Verification items for this drawing (mm, ordinates from the low corner). Round coordinates to 2 decimals unless told otherwise and drop trailing zeros. Order: outer loops, then holes, each group sorted by start corner. A loop starts at its lowest first (then second) coordinate and runs counter-clockwise, first axis right, second up. Notation, with made-up numbers: (25, -6.5) -> (49, -6.5) arc R16 cw to (49, 1.5) -> close; hole circle Ø10 at (44.25, 42). An arc over 180 degrees is marked (long way). Return JSON: item names as keys, results as strings. Group by question number.
Item 1: Draft check along Y on the marked faces 1, 2 and 3. Enter one of: pulls with the +Y half, pulls with the -Y half, needs draft (parallel to the pull), parting line crosses it, or undercut.
Item 2: Scan lines: probe 1 along Y at (x, z) = (12.7, 6.25); probe 2 along Z at (x, y) = (10.5, 2.25); probe 3 along X at (y, z) = (8.5, 7) (1 decimal). Record each from-to range of solid material in increasing order. Write a range as from..to.
Item 3: Sectioned sample at B-B on y = 8.5. Record the cut outline in (x, z) (1 decimal).
Item 4: Depth check by flat-ended pin: pin 1 Ø5 at (y, z) = (14, 5) entering from +X; pin 2 Ø1.5 at (x, y) = (19, 6) entering from +Z. Enter the tip coordinate at first touch or a pass-through.
Item 5: Sectioned sample at A-A on x = 12.7. Record the cut outline in (y, z).
Item 6: Sectioned sample at C-C on z = 2.5. Record the cut outline in (x, y).
Item 7: Sectioned sample at D-D on y = 6.25. Record the cut outline in (x, z).
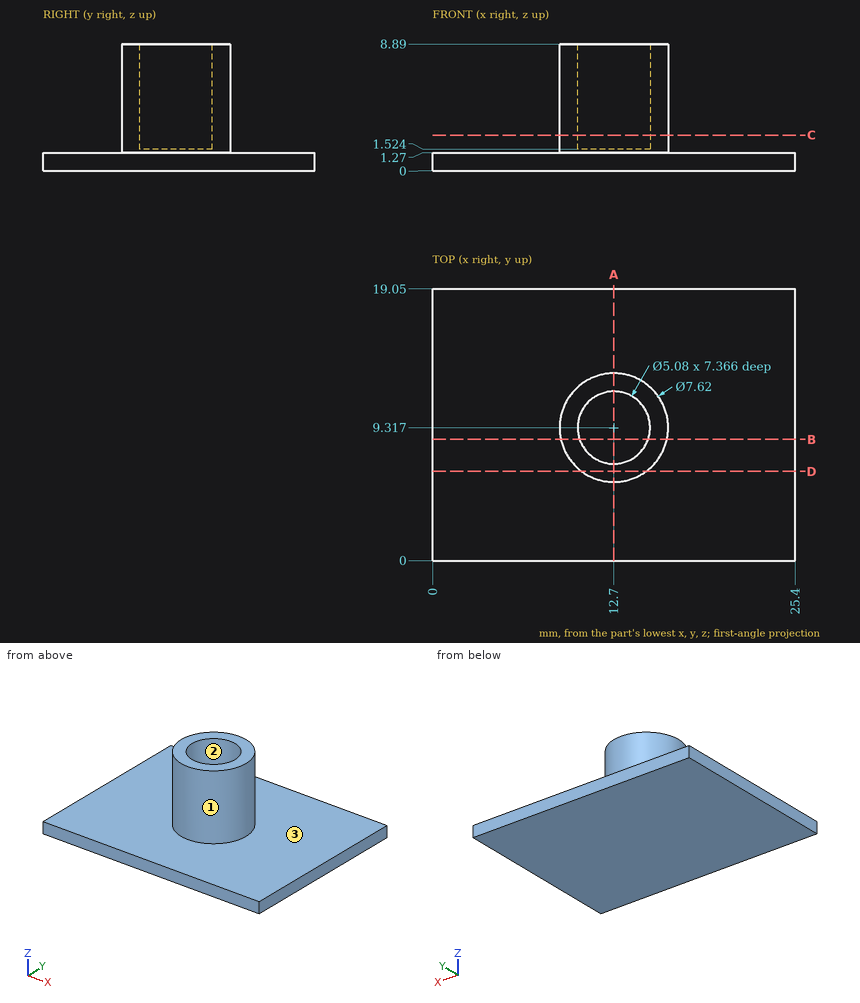
Recorded:
{
 "1": {"face 1": "parting line crosses it", "face 2": "undercut", "face 3": "needs draft"},
 "2": {"probe 1": "5.51..6.78, 11.86..13.13", "probe 2": "0..1.27", "probe 3": "9..10.3, 15.1..16.4"},
 "3": {"outline": "(0, 0) -> (25.4, 0) -> (25.4, 1.3) -> (16.4, 1.3) -> (16.4, 8.9) -> (15.1, 8.9) -> (15.1, 1.5) -> (10.3, 1.5) -> (10.3, 8.9) -> (9, 8.9) -> (9, 1.3) -> (0, 1.3) -> close"},
 "4": {"pin 1": "x = 15.82", "pin 2": "z = 1.27"},
 "5": {"outline": "(0, 0) -> (19.05, 0) -> (19.05, 1.27) -> (13.13, 1.27) -> (13.13, 8.89) -> (11.86, 8.89) -> (11.86, 1.52) -> (6.78, 1.52) -> (6.78, 8.89) -> (5.51, 8.89) -> (5.51, 1.27) -> (0, 1.27) -> close"},
 "6": {"outline": "circle Ø7.62 at (12.7, 9.32); hole circle Ø5.08 at (12.7, 9.32)"},
 "7": {"outline": "(0, 0) -> (25.4, 0) -> (25.4, 1.27) -> (14.96, 1.27) -> (14.96, 8.89) -> (10.44, 8.89) -> (10.44, 1.27) -> (0, 1.27) -> close"}
}
